from build123d import *

# Parameters (mm, degrees)
SKETCH_1_W      = 33
SKETCH_1_H      = 16
SKETCH_1_R      = 1.75
EXTRUDE_1_DEPTH = 1
SKETCH_2_W      = 3
SKETCH_2_H      = 2
EXTRUDE_2_DEPTH = 3


with BuildPart() as part:
    # Эскиз1 → Бобышка-Вытянуть1 (new body)
    with BuildSketch(Plane(origin=(0, 0, 0), x_dir=(1, 0, 0), z_dir=(0, 1, 0))):
        with Locations((-16.5, 0)):
            Rectangle(SKETCH_1_W, SKETCH_1_H)
        with Locations(Location((-16.5, 0, 0), (0, 0, 270))):
            Circle(SKETCH_1_R, mode=Mode.SUBTRACT)
    extrude(amount=EXTRUDE_1_DEPTH)

    # Эскиз2 → Бобышка-Вытянуть2 (add)
    with BuildSketch(Plane(origin=(0, 0, 0), x_dir=(1, 0, 0), z_dir=(0, 1, 0))):
        with Locations((-24.5, -3.674415698)):
            Rectangle(SKETCH_2_W, SKETCH_2_H)
    extrude(amount=EXTRUDE_2_DEPTH)


solid = part.part
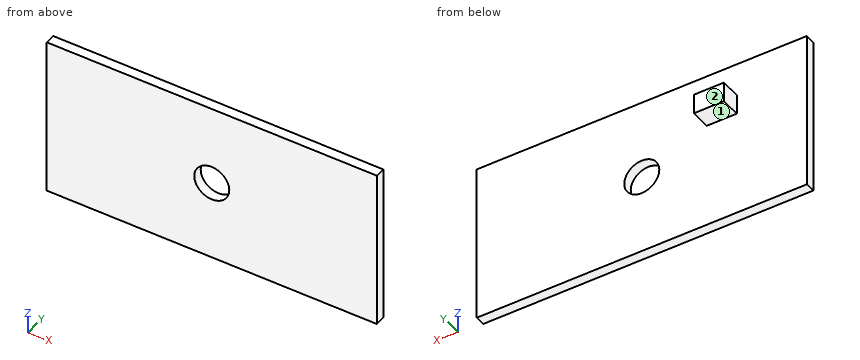
Build history of the part. All positions in model axes, mm. Face numbers are marked on the shaded views. A direction names the side the tool comes from. Round coordinates to 2 decimals unless told otherwise and drop trailing zeros. Loops run counter-clockwise (first coordinate to the right, second up) from the corner with the lowest first, then second, coordinate; pieces in that order, holes last. Notation, with made-up numbers: (71.25, 39) -> (86.25, 39) arc R12 cw to (86.25, 55) -> close; hole circle Ø1 at (79.5, 26.5). An arc over 180 degrees is marked (long way). Answer in a Markdown table with one row per item.
Item 1: Saw through at B-B (z = 0). Write the cut outline in (x, y), and give its area (3 significant figures).
Answers below:
| item | result |
|---|---|
| outline | (-33, 0) -> (-18.25, 0) -> (-18.25, 1) -> (-33, 1) -> close; (-14.75, 0) -> (0, 0) -> (0, 1) -> (-14.75, 1) -> close |
| area | 29.5 mm² |
Item 2: Saw through at D-D (x = -6.5). Write the cut outline in (y, z), and give its area (3 significant figures).
Answers below:
| item | result |
|---|---|
| outline | (0, -8) -> (1, -8) -> (1, 8) -> (0, 8) -> close |
| area | 16.0 mm² |
Item 3: Saw through at C-C (z = 4). Write the cut outline in (x, y), and give its area (3 significant figures).
Answers below:
| item | result |
|---|---|
| outline | (-33, 0) -> (0, 0) -> (0, 1) -> (-23, 1) -> (-23, 3) -> (-26, 3) -> (-26, 1) -> (-33, 1) -> close |
| area | 39.0 mm² |
Item 4: Drill centre lines: L1, parallel to X at y = 0.2, z = 0; L2, parallel to Y at x = -5.5, z = -4.5; L3, parallel to X at y = 0.95, z = -1. Where is each one in solid material? Low to high. Write a range as [from, to].
Answers below:
| item | result |
|---|---|
| L1 | x = [-33, -18.25], [-14.75, 0] |
| L2 | y = [0, 1] |
| L3 | x = [-33, -17.94], [-15.06, 0] |
Item 5: Which spindle directions (+Z, -Z, +X, -X, +Y, -Y) get a long thin tool onto all of the face, cutting with end or side? Do the marked faces 1 and 2. Say none if no direction does.
Answers below:
| item | result |
|---|---|
| face 1 | -Z, +X, -X, +Y |
| face 2 | +Z, -Z, +X, -X, +Y |
Item 6: Pin check, flat tips, straight feed: pin 1 (5 mm diameter, centred on x = -21.5, z = -1, fed in from +Y); pin 2 (0.6 mm diameter, centred on x = -25, y = 2, fed in from +Z); pin 3 (1 mm diameter, centred on y = 2, z = 3.5, fed in from -X). Stop position of each tip, or through.
Answers below:
| item | result |
|---|---|
| pin 1 | stops at y = 1 |
| pin 2 | stops at z = 4.67 |
| pin 3 | stops at x = -26 |
Item 7: Saw through at A-A (x = -16.5). Write the cut outline in (y, z), and give its area (3 significant figures).
Answers below:
| item | result |
|---|---|
| outline | (0, -8) -> (1, -8) -> (1, -1.75) -> (0, -1.75) -> close; (0, 1.75) -> (1, 1.75) -> (1, 8) -> (0, 8) -> close |
| area | 12.5 mm² |
